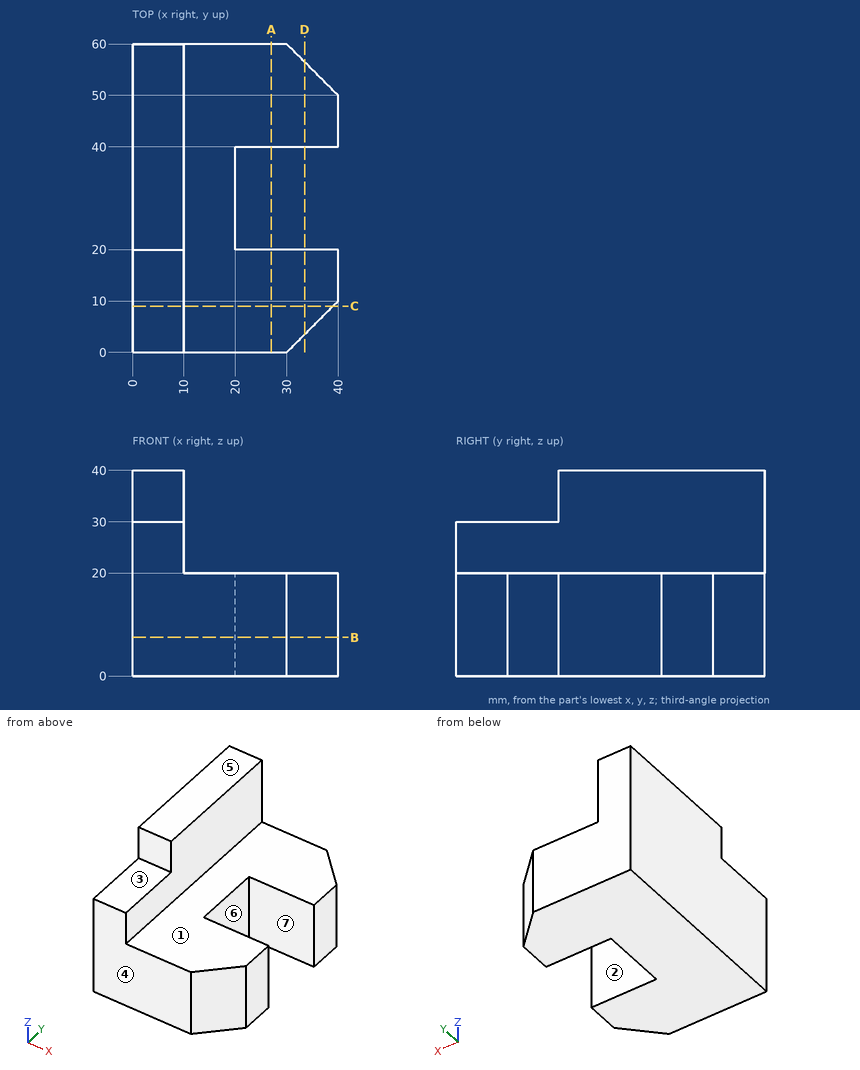
Check sheet for the drawn part. Datum: minimum x, y, z corner. Units: mm. A direction names the side the tool comes from. Round coordinates to 2 decimals unless told otherwise and drop trailing zeros. Order: outer loops, then holes, each group sorted by start corner. A loop starts at its lowest first (then second) coordinate and runs counter-clockwise, first axis right, second up. Notation, with made-up numbers: M 15,83 L 66,83 A17 ccw 66,113 Z; hole C 43.5,45.25 d11. An arc over 180 degrees is marked long. Write each question's results on one line, items separated by ' | '. Start each with the question number.
1. Go/stop test with flat-tipped pins: P1, Ø8, axis at x = 7, y = 12, coming from the +Z side; P2, Ø10, axis at x = 28.5, y = 9, coming from the +Z side; P3, Ø4, axis at y = 52, z = 24.5, coming from the +X side. Record where each tip stops, or that it passes through.
2. Cross-section at B-B on z = 7.5. Record the boundary of the cut face in (x, y).
3. Material ranges on L1, parallel to Y at x = 30, z = 5.5; L2, parallel to X at y = 52.5, z = 25.5; L3, parallel to Z at x = 8.5, y = 4, recorded low to high. Write a range as from..to.
4. Cross-section at D-D on x = 33.5. Record the boundary of the cut face in (y, z).
5. Set-up check for the marked faces 1, 2 and 3: record each of +Z, -Z, +X, -X, +Y, -Y from which the full face is reachable in a straight line by a thin tool's end or side.
6. Cross-section at A-A on x = 27. Record the boundary of the cut face in (y, z).
7. Cross-section at C-C on y = 9. Record the boundary of the cut face in (x, z).
8. Draft check along Y on the marked faces 4, 5, 6 and 7. Enter one of: pulls with the +Y half, pulls with the -Y half, needs draft (parallel to the pull), parting line crosses it, or undercut.
Resolved:
1) P1: z = 30 | P2: z = 20 | P3: x = 10
2) outline: M 0,0 L 30,0 L 40,10 L 40,20 L 20,20 L 20,40 L 40,40 L 40,50 L 30,60 L 0,60 Z
3) L1: 0..20, 40..60 | L2: 0..10 | L3: 0..30
4) outline: M 3.5,0 L 20,0 L 20,20 L 3.5,20 Z; M 40,0 L 56.5,0 L 56.5,20 L 40,20 Z
5) face 1: +Z, +X, +Y, -Y | face 2: +Z, -Z, +X | face 3: +Z, +X, -X, -Y
6) outline: M 0,0 L 20,0 L 20,20 L 0,20 Z; M 40,0 L 60,0 L 60,20 L 40,20 Z
7) outline: M 0,0 L 39,0 L 39,20 L 10,20 L 10,30 L 0,30 Z
8) face 4: pulls with the -Y half | face 5: needs draft | face 6: undercut | face 7: undercut
